Geometry check sheet. Reference: drawing and pictorial views, mm from the part's lowest x, y, z. A direction names the side the tool comes from. Round coordinates to 2 decimals unless told otherwise and drop trailing zeros. Loops run counter-clockwise (first coordinate to the right, second up) from the corner with the lowest first, then second, coordinate; pieces in that order, holes last. Notation, with made-up numbers: (-13, 63) - (44, 63) arc R22 ccw to (44, 85) - close; hole circle Ø1 at (77.5, 57.25). An arc over 180 degrees is marked (long way). Answer in a Markdown table with one row per item. Add a question column.
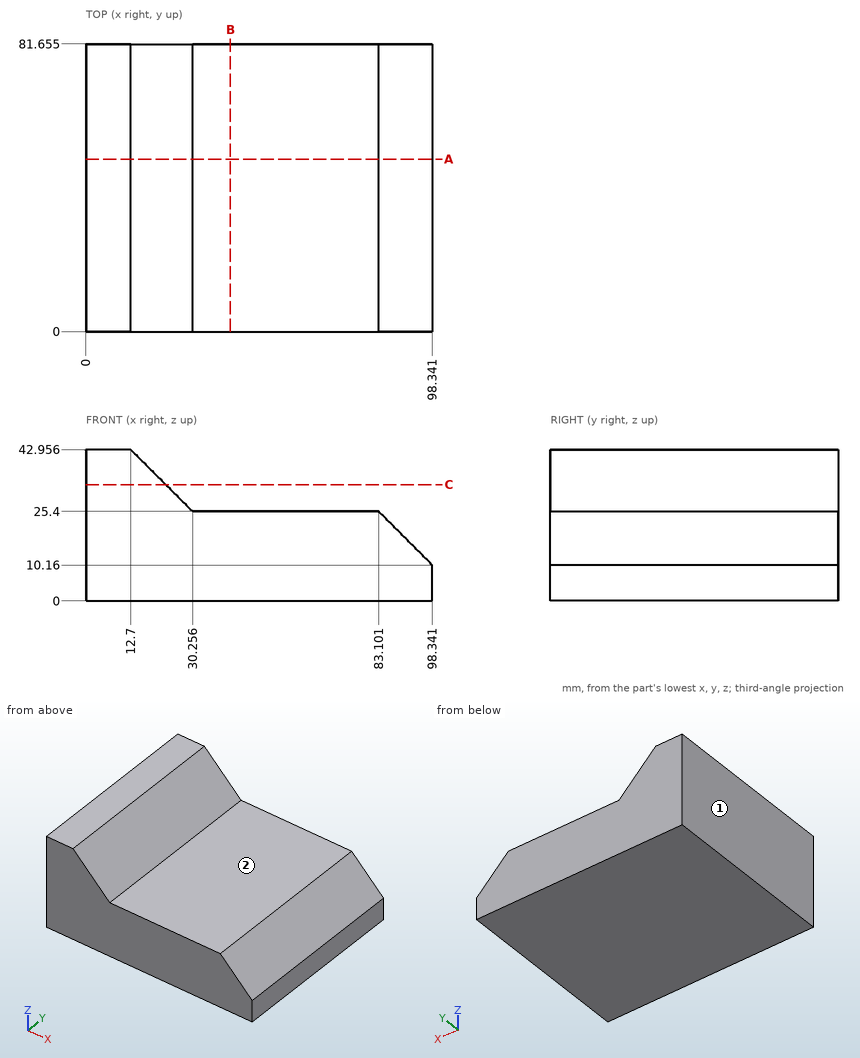
Q1. Depth check by flat-ended pin: P1, Ø3, axis at x = 21.5, y = 17, coming from the +Z side (1 decimal); P2, Ø4, axis at x = 51.5, y = 69, coming from the -Z side; P3, Ø4, axis at y = 41.5, z = 37.5, coming from the +X side (1 decimal); P4, Ø8, axis at x = 57.5, y = 23.5, coming from the +Z side. Enter the tip coordinate at first touch or a pass-through.
Q2. Scan lines: line 1 (Z direction, x = 59.5, y = 48); line 2 (X direction, y = 56.5, z = 29.5) (1 decimal); line 3 (X direction, y = 62.5, z = 16). Record each from-to range of solid material in increasing order. Write a range as from..to.
Q3. Cross-section at A-A, the plane y = 49. Enter the section's corners in (x, z) (1 decimal), plus the area to 3 significant figures.
Q4. Cross-section at B-B, the plane x = 41. Enter the section's corners in (y, z) (1 decimal), plus the area to 3 significant figures.
Q5. Cross-section at C-C, the plane z = 33. Enter the section's corners in (x, y) (1 decimal), plus the area to 3 significant figures.
Q6. Set-up check for the marked faces 1 and 2: record each of +Z, -Z, +X, -X, +Y, -Y from which the full face is reachable in a straight line by a thin tool's end or side.
Check sheet entries:
| question | item | result |
|---|---|---|
| 1 | P1 | z = 35.7 |
| 1 | P2 | z = 0 |
| 1 | P3 | x = 20.2 |
| 1 | P4 | z = 25.4 |
| 2 | line 1 | 0..25.4 |
| 2 | line 2 | 0..26.2 |
| 2 | line 3 | 0..92.5 |
| 3 | outline | (0, 0) - (98.3, 0) - (98.3, 10.2) - (83.1, 25.4) - (30.3, 25.4) - (12.7, 43) - (0, 43) - close |
| 3 | area | 2,760 mm² |
| 4 | outline | (0, 0) - (81.7, 0) - (81.7, 25.4) - (0, 25.4) - close |
| 4 | area | 2,070 mm² |
| 5 | outline | (0, 0) - (22.7, 0) - (22.7, 81.7) - (0, 81.7) - close |
| 5 | area | 1,850 mm² |
| 6 | face 1 | +Z, -Z, -X, +Y, -Y |
| 6 | face 2 | +Z, +X, +Y, -Y |
